Part model, mm, in its own coordinate system. A direction names the side the tool comes from. Round coordinates to 2 decimals unless told otherwise and drop trailing zeros. Write each loop counter-clockwise with the first axis right and the second up, starting at its lowest first coordinate (ties: lowest second). Pieces come first, ordered by that corner, then holes. Notation, with made-up numbers: (0.5, 22) -> (56.5, 22) arc R13 cw to (56.5, 31) -> close; hole circle Ø9 at (-22.5, -3). An arc over 180 degrees is marked (long way). Use CSV: the item, a comma, the result in double quotes. Start each with the question number.
```python
from build123d import *

# Parameters (mm, degrees)
F1_DEPTH  = 18
F3_D      = 3.2
F3_DEPTH  = 15
F4_W      = 6
F4_H      = 6
F5_DEPTH  = 10
F6_W      = 6
F6_H      = 6
F7_DEPTH  = 10
F9_D      = 3.2
F9_DEPTH  = 6
F11_D     = 3.2
F11_DEPTH = 6


with BuildPart() as f1:
    # F0 (on Top) → F1 (new body)
    with BuildSketch(Plane.XY):
        with BuildLine():
            Line((3, 13.278079), (-14.3, 13.278079))
            Line((-14.3, 13.278079), (-14.3, 10.278079))
            Line((-14.3, 10.278079), (0.622289, 10.278079))
            ThreePointArc((0.622289, 10.278079), (11.5, 2.620549), (22.377711, 10.278079))
            Line((22.377711, 10.278079), (23, 10.278079))
            Line((23, 10.278079), (37.3, 10.278079))
            Line((37.3, 10.278079), (37.3, 17.778079))
            Line((37.3, 17.778079), (22.406277, 17.778079))
            ThreePointArc((22.406277, 17.778079), (11.5, 25.549511), (0.593723, 17.778079))
            Line((0.593723, 17.778079), (-14.3, 17.778079))
            Line((-14.3, 17.778079), (-14.3, 14.778079))
            Line((-14.3, 14.778079), (3, 14.778079))
            ThreePointArc((3, 14.778079), (11.5, 22.528734), (20, 14.778079))
            Line((20, 14.778079), (25.6, 14.778079))
            Line((25.6, 14.778079), (25.6, 13.278079))
            Line((25.6, 13.278079), (23, 13.278079))
            Line((23, 13.278079), (20, 13.278079))
            ThreePointArc((20, 13.278079), (11.5, 5.523889), (3, 13.278079))
        make_face()
    extrude(amount=F1_DEPTH)

    # F3
    with Locations(Plane.XZ.offset(-10.278079)):
        with Locations((-6.838855, 9)):
            Hole(F3_D / 2, depth=F3_DEPTH)

    # F4 (on face) → F5 (join)
    with BuildSketch(Plane.XZ.offset(-10.278079)):
        with Locations((34.3, 3)):
            Rectangle(F4_W, F4_H)
    extrude(amount=F5_DEPTH)

    # F6 (on face) → F7 (join)
    with BuildSketch(Plane.XZ.offset(-10.278079)):
        with Locations((-11.3, 3)):
            Rectangle(F6_W, F6_H)
    extrude(amount=F7_DEPTH)

    # F9
    with Locations(Plane.YZ.offset(37.3)):
        with Locations((3.748374, 3)):
            Hole(F9_D / 2, depth=F9_DEPTH)

    # F11
    with Locations(Plane(origin=(-14.3, 0, 0), x_dir=(0, -1, 0), z_dir=(-1, 0, 0))):
        with Locations((-3.278079, 3)):
            Hole(F11_D / 2, depth=F11_DEPTH)


solid = f1.part
```
1. Band-saw the part on A-A (x = -9). List the corners of the cut face in (y, z), then the cut area to 3 significant figures.
2. Which spindle directions (+Z, -Z, +X, -X, +Y, -Y) get a long thin tool onto all of the face, cutting with end or side? Do faces 4 (the flat face through (31.3, 5.35, 2.29)), 5 (the flat face through (34, 5, 6)), 6 (the flat face through (-5, 17.778, 9)). Say none if no direction does.
3. Flat gauge pins, fed straight in: pin 1 (1.8 mm diameter, centred on x = 35, y = 6.5, fed in from +Z); pin 2 (1 mm diameter, centred on y = 3, z = 7.5, fed in from +X); pin 3 (2 mm diameter, centred on x = 15.5, z = 12, fed in from -Y); pin 4 (5 mm diameter, centred on y = 3.75, z = 3, fed in from +X). Where does each tip first touch, or does it go through?
4. Band-saw the part on C-C (y = 16.75). List the corners of the cut face in (x, z), then the cut area to 3 significant figures.
5. Band-saw the part on B-B (z = 3). List the corners of the cut face in (x, y).
6. Pull direction Y, two halves, no side cores. Call faces 1 (the cylindrical face through (-6.49, 11.8, 7.44)), 2 (the cylindrical face through (11.677, 5.526, 8.874)), 3 (the cylindrical face through (11.302, 2.622, 8.874)): released by +Y, released by -Y, zero draft, split by the parting line, or undercut.
7. Drill centre lines: line 1 along X through (y, z) = (5.25, 5.25); line 2 along Y through (x, z) = (16, 11.5); line 3 along Y through (x, z) = (6, 6). Where is each one in solid material? Low to high. Write a range as [from, to].
8. Band-saw the part on D-D (y = 7). List the corners of the cut face in (x, z).
Answers below:
1,outline,"(0.28, 0) -> (13.28, 0) -> (13.28, 18) -> (10.28, 18) -> (10.28, 6) -> (0.28, 6) -> close; (14.78, 0) -> (17.78, 0) -> (17.78, 18) -> (14.78, 18) -> close; hole circle Ø3.2 at (3.28, 3)"
1,area,"160 mm^2"
2,face 4,"+Z, -Z, -Y"
2,face 5,"+Z, +X, -Y"
2,face 6,"+Z, -Z, -X, +Y"
3,pin 1,"stops at z = 6"
3,pin 2,"stops at x = 15.92"
3,pin 3,"stops at y = 3.02"
3,pin 4,"stops at x = 37.3"
4,outline,"(-14.3, 0) -> (3.42, 0) -> (3.42, 18) -> (-14.3, 18) -> close; (19.58, 0) -> (37.3, 0) -> (37.3, 18) -> (19.58, 18) -> close; hole circle Ø3.2 at (-6.84, 9)"
4,area,"630 mm^2"
5,outline,"(-14.3, 0.28) -> (-8.3, 0.28) -> (-8.3, 1.68) -> (-14.3, 1.68) -> close; (-14.3, 4.88) -> (-8.3, 4.88) -> (-8.3, 10.28) -> (0.62, 10.28) arc R11.55 ccw to (22.38, 10.28) -> (31.3, 10.28) -> (31.3, 5.35) -> (37.3, 5.35) -> (37.3, 17.78) -> (22.41, 17.78) arc R11.54 ccw to (0.59, 17.78) -> (-14.3, 17.78) -> (-14.3, 14.78) -> (3, 14.78) arc R8.54 cw to (20, 14.78) -> (25.6, 14.78) -> (25.6, 13.28) -> (20, 13.28) arc R8.54 cw to (3, 13.28) -> (-14.3, 13.28) -> close; (31.3, 0.28) -> (37.3, 0.28) -> (37.3, 2.15) -> (31.3, 2.15) -> close"
6,face 1,"zero draft"
6,face 2,"undercut"
6,face 3,"released by -Y"
7,line 1,"x = [-14.3, -8.3], [4.16, 18.84], [31.3, 37.3]"
7,line 2,"y = [3.53, 6.81], [21.25, 24.64]"
7,line 3,"y = [4.01, 7.53], [20.52, 24.15]"
8,outline,"(-14.3, 0) -> (-8.3, 0) -> (-8.3, 6) -> (-14.3, 6) -> close; (2.44, 0) -> (6.7, 0) -> (6.7, 18) -> (2.44, 18) -> close; (16.3, 0) -> (20.56, 0) -> (20.56, 18) -> (16.3, 18) -> close; (31.3, 0) -> (37.3, 0) -> (37.3, 6) -> (31.3, 6) -> close"
